```python
from build123d import *

# Parameters (mm, degrees)
SKETCH1_W                  = 60
SKETCH1_H                  = 50
BOSS_EXTRUDE1_DEPTH        = 6.35
CUT_EXTRUDE1_DEPTH         = 40.564156758
CUT_EXTRUDE2_DEPTH         = 40.564156758
HOLE1_D                    = 25
F_2_CLEARANCE_HOLE1_REACH  = 60.654
F_2_CLEARANCE_HOLE1_BORE_R = 1.25
F_8_CLEARANCE_HOLE1_D      = 4.499991
CHAMFER1_SIZE              = 2.449999926


with BuildPart() as part:
    # Sketch1 → Boss-Extrude1 (new body)
    with BuildSketch(Plane(origin=(0, 0, 0), x_dir=(-1, 0, 0), z_dir=(0, 0, -1))):
        Rectangle(SKETCH1_W, SKETCH1_H)
    extrude(amount=-BOSS_EXTRUDE1_DEPTH)

    # Sketch2 → Cut-Extrude1 (cut, through all)
    with BuildSketch(Plane(origin=(0, 0, 0), x_dir=(-1, 0, 0), z_dir=(0, 0, -1))):
        with BuildLine():
            Line((23.25, 19), (23.25, -17))
            ThreePointArc((23.25, -17), (25.5, -19.25), (27.75, -17))
            Line((27.75, -17), (27.75, 19))
            ThreePointArc((27.75, 19), (25.5, 21.25), (23.25, 19))
        make_face()
    extrude(amount=-CUT_EXTRUDE1_DEPTH, mode=Mode.SUBTRACT)

    # Sketch3 → Cut-Extrude2 (cut, through all)
    with BuildSketch(Plane.XY.offset(6.35)):
        with BuildLine():
            Line((27.75, -17), (27.75, 19))
            ThreePointArc((27.75, 19), (25.5, 21.25), (23.25, 19))
            Line((23.25, 19), (23.25, -17))
            ThreePointArc((23.25, -17), (25.5, -19.25), (27.75, -17))
        make_face()
    extrude(amount=-CUT_EXTRUDE2_DEPTH, mode=Mode.SUBTRACT)

    # Hole1 (through all)
    with Locations(Plane(origin=(0, 0, 0), x_dir=(-1, 0, 0), z_dir=(0, 0, -1))):
        with Locations((0, 0)):
            Hole(HOLE1_D / 2)

    # #2 Clearance Hole1 bore → #2 Clearance Hole1 (cut, up to next)
    with BuildSketch(Plane(origin=(0, -25, 0), x_dir=(-1, 0, 0), z_dir=(0, -1, 0)), mode=Mode.PRIVATE) as f_2_clearance_hole1_sk1:
        with Locations((-25.5, -3.175)):
            Circle(F_2_CLEARANCE_HOLE1_BORE_R)
    f_2_clearance_hole1_tool1 = extrude(f_2_clearance_hole1_sk1.sketch, amount=-F_2_CLEARANCE_HOLE1_REACH, mode=Mode.PRIVATE) & part.part
    # #2 Clearance Hole1 bore → #2 Clearance Hole1 (cut, up to next)
    with BuildSketch(Plane(origin=(0, -25, 0), x_dir=(-1, 0, 0), z_dir=(0, -1, 0)), mode=Mode.PRIVATE) as f_2_clearance_hole1_sk2:
        with Locations((25.5, -3.175)):
            Circle(F_2_CLEARANCE_HOLE1_BORE_R)
    f_2_clearance_hole1_tool2 = extrude(f_2_clearance_hole1_sk2.sketch, amount=-F_2_CLEARANCE_HOLE1_REACH, mode=Mode.PRIVATE) & part.part
    add(f_2_clearance_hole1_tool1.solids().sort_by_distance((25.5, -25, 3.175))[0], mode=Mode.SUBTRACT)
    add(f_2_clearance_hole1_tool2.solids().sort_by_distance((-25.5, -25, 3.175))[0], mode=Mode.SUBTRACT)

    # #8 Clearance Hole1 (through all)
    with Locations(Plane(origin=(0, 0, 0), x_dir=(-1, 0, 0), z_dir=(0, 0, -1))):
        with Locations((-12.374368671, 12.374368671), (-12.374368671, -12.374368671), (12.374368671, -12.374368671), (12.374368671, 12.374368671)):
            Hole(F_8_CLEARANCE_HOLE1_D / 2)

    # Chamfer1
    chamfer1_edges = [part.edges().sort_by_distance(p)[0] for p in [
        (-14.624364171, 12.374368671, 6.35),
        (-14.624364171, -12.374368671, 6.35),
        (10.124373171, -12.374368671, 6.35),
        (10.124373171, 12.374368671, 6.35),
    ]]
    chamfer(chamfer1_edges, length=CHAMFER1_SIZE)


solid = part.part
```
Could you check a few things on this model? Use its own coordinates, in mm. A direction names the side the tool comes from. Give positions to 0.01 mm unless a question says otherwise; leave off trailing zeros. Loops run counter-clockwise (first coordinate to the right, second up) from the corner with the lowest first, then second, coordinate; pieces in that order, holes last. Notation, with made-up numbers: (77.5, -27) - (88.5, -27) arc R10 ccw to (88.5, -22) - close; hole circle Ø10 at (79.5, 31). An arc over 180 degrees is marked (long way). Use one line per item in the form item = value.
1. I want a section at D-D (y = 20). Please give me the cut outline in (x, z), and give its area (3 significant figures).
Response values:
outline = (-30, 0) - (-27.52, 0) - (-27.52, 6.35) - (-30, 6.35) - close; (-23.48, 0) - (23.48, 0) - (23.48, 6.35) - (-23.48, 6.35) - close; (27.52, 0) - (30, 0) - (30, 6.35) - (27.52, 6.35) - close
area = 330 mm²
2. I'm going to push flat-ended pins straight in: pin 1 Ø2 at (x, z) = (-25.5, 3.175) entering from -Y; pin 2 Ø1.5 at (x, z) = (25.5, 3.175) entering from -Y; pin 3 Ø6 at (x, y) = (-12.37, -12.37) entering from +Z. Where does each tip first touch, or does it pass through?
Response values:
pin_1 = 21.02
pin_2 = 21.12
pin_3 = 4.66
3. I want a section at C-C (x = 0). Please give me the cut outline in (y, z), and give its area (3 significant figures).
Response values:
outline = (-25, 0) - (-12.5, 0) - (-12.5, 6.35) - (-25, 6.35) - close; (12.5, 0) - (25, 0) - (25, 6.35) - (12.5, 6.35) - close
area = 159 mm²
4. I want a section at A-A (x = -25.5). Please give me the cut outline in (y, z) (3 decimals).
Response values:
outline = (-25, 0) - (-19.25, 0) - (-19.25, 1.925) - (-25, 1.925) - close; (-25, 4.425) - (-19.25, 4.425) - (-19.25, 6.35) - (-25, 6.35) - close; (21.25, 0) - (25, 0) - (25, 6.35) - (21.25, 6.35) - close
5. I need wall thicknesses on probe 1 along X at (y, z) = (19, 4.25); probe 2 along X at (y, z) = (-6.5, 5.5). Which ranges of each line are inside material? Lowest first, please.
Response values:
probe_1 = -30 to -27.75, -23.25 to 23.25, 27.75 to 30
probe_2 = -30 to -27.75, -23.25 to -10.68, 10.68 to 23.25, 27.75 to 30
6. Thinking about a two-plate mould opening in Y: for faces 1 (the face through (0, -25, 3)), 2 (the face through (-26.655, -21.978, 3.654)), 3 (the face through (11.923, 3.755, 3.219)), which applies, released by +Y, released by -Y, zero draft, split by the parting line, or undercut?
Response values:
face_1 = released by -Y
face_2 = zero draft
face_3 = undercut
7. On a 3-axis mill with a long thin cutter (end or side, diameter ignored), from which of +Z, -Z, +X, -X, +Y, -Y can I reach the whole of each face in a straight line? I mean faces 4 (the face through (24.345, -21.978, 3.654)), 5 (the face through (10.008, -12.27, 4.019)), 6 (the face through (23.25, 1, 3)). Say none if no direction works.
Response values:
face_4 = -Y
face_5 = +Z
face_6 = +Z, -Z
8. I want a section at B-B (y = 0). Please give me the cut outline in (x, z).
Response values:
outline = (-30, 0) - (-27.75, 0) - (-27.75, 6.35) - (-30, 6.35) - close; (-23.25, 0) - (-12.5, 0) - (-12.5, 6.35) - (-23.25, 6.35) - close; (12.5, 0) - (23.25, 0) - (23.25, 6.35) - (12.5, 6.35) - close; (27.75, 0) - (30, 0) - (30, 6.35) - (27.75, 6.35) - close
